Verification items for the finished model (mm, model axes). A direction names the side the tool comes from. Coordinates: 2 decimals unless noted, no trailing zeros. Write each loop counter-clockwise with the first axis right and the second up, starting at its lowest first coordinate (ties: lowest second). Pieces come first, ordered by that corner, then holes. Notation, with made-up numbers: (-12.75, 87.25) -> (35.25, 87.25) arc R27 cw to (35.25, 103.25) -> close; hole circle Ø6 at (9, 6). An arc over 180 degrees is marked (long way). Use CSV: the item, a comma, the result in double quotes.
```python
from build123d import *

# Parameters (mm, degrees)
F1_DEPTH = 30
F3_DEPTH = 84.001
F4_R     = 3
F5_DEPTH = 50.001


with BuildPart() as f1:
    # F0 (on Top) → F1 (new body)
    with BuildSketch(Plane.XY):
        with BuildLine():
            Line((0, 45), (0, 0))
            Line((0, 0), (2, 0))
            Line((2, 0), (2, 43))
            ThreePointArc((2, 43), (3.464466, 46.535534), (7, 48))
            Line((7, 48), (77, 48))
            ThreePointArc((77, 48), (80.535534, 46.535534), (82, 43))
            Line((82, 43), (82, 0))
            Line((82, 0), (84, 0))
            Line((84, 0), (84, 45))
            ThreePointArc((84, 45), (82.535534, 48.535534), (79, 50))
            Line((79, 50), (5, 50))
            ThreePointArc((5, 50), (1.464466, 48.535534), (0, 45))
        make_face()
    extrude(amount=F1_DEPTH)

    # F2 (on face) → F3 (cut, through all)
    with BuildSketch(Plane(origin=(0, 0, 0), x_dir=(0, -1, 0), z_dir=(-1, 0, 0))):
        with BuildLine():
            Line((-10, 18), (-30, 18))
            ThreePointArc((-30, 18), (-33, 15), (-30, 12))
            Line((-30, 12), (-10, 12))
            ThreePointArc((-10, 12), (-7, 15), (-10, 18))
        make_face()
    extrude(amount=-F3_DEPTH, mode=Mode.SUBTRACT)

    # F4 (on face) → F5 (cut, through all)
    with BuildSketch(Plane(origin=(0, 50, 0), x_dir=(-1, 0, 0), z_dir=(0, 1, 0))):
        with Locations((-68.6, 15)):
            Circle(F4_R)
        with Locations((-15.4, 15)):
            Circle(F4_R)
    extrude(amount=-F5_DEPTH, mode=Mode.SUBTRACT)


solid = f1.part
```
1) Cross-section at C-C (y = 15). Record the boundary of the cut face in (x, z), plus the area to 3 significant figures.
Return value:
outline,"(0, 0) -> (2, 0) -> (2, 12) -> (0, 12) -> close; (0, 18) -> (2, 18) -> (2, 30) -> (0, 30) -> close; (82, 0) -> (84, 0) -> (84, 12) -> (82, 12) -> close; (82, 18) -> (84, 18) -> (84, 30) -> (82, 30) -> close"
area,"96.0 mm2"
2) Mould release check, pull along Z, two halves, no side actions. Record for faces 4 (the flat face through (42, 49, 0)), 5 (the cylindrical face through (80, 47, 15)), 6 (the cylindrical face through (16.05, 49.01, 12.07)): released by +Z, released by -Z, zero draft, split by the parting line, or undercut.
Return value:
face 4,"released by -Z"
face 5,"zero draft"
face 6,"undercut"
3) Cross-section at B-B (x = 68.6). Record the boundary of the cut face in (y, z), plus the area to 3 significant figures.
Return value:
outline,"(48, 0) -> (50, 0) -> (50, 12) -> (48, 12) -> close; (48, 18) -> (50, 18) -> (50, 30) -> (48, 30) -> close"
area,"48.0 mm2"
4) Scan lines: L1, parallel to X at y = 19, z = 10.75; L2, parallel to Z at x = 15.4, y = 49.05; L3, parallel to Y at x = 67, z = 23.5. Record each from-to range of solid material in increasing order.
Return value:
L1,"0 to 2, 82 to 84"
L2,"0 to 12, 18 to 30"
L3,"48 to 50"
5) Cross-section at A-A (y = 36). Record the boundary of the cut face in (x, z).
Return value:
outline,"(0, 0) -> (2, 0) -> (2, 30) -> (0, 30) -> close; (82, 0) -> (84, 0) -> (84, 30) -> (82, 30) -> close"
6) Cross-section at D-D (z = 23.5). Record the boundary of the cut face in (x, y).
Return value:
outline,"(0, 0) -> (2, 0) -> (2, 43) arc R5 cw to (7, 48) -> (77, 48) arc R5 cw to (82, 43) -> (82, 0) -> (84, 0) -> (84, 45) arc R5 ccw to (79, 50) -> (5, 50) arc R5 ccw to (0, 45) -> close"
7) Gauge pin test, flat end, axial feed: pin 1 (5 mm diameter, centred on x = 74, z = 5.5, fed in from -Y). Record the tip position at first contact, or that the pin passes through.
Return value:
pin 1,"y = 48"
8) Set-up check for faces 1 (the flat face through (42, 48, 15)), 2 (the cylindrical face through (71, 49, 13.2)), 3 (the cylindrical face through (83, 7, 15)): record each of +Z, -Z, +X, -X, +Y, -Y from which the full face is reachable in a straight line by a thin tool's end or side.
Return value:
face 1,"+Z, -Z, -Y"
face 2,"+Y, -Y"
face 3,"+X, -X"
